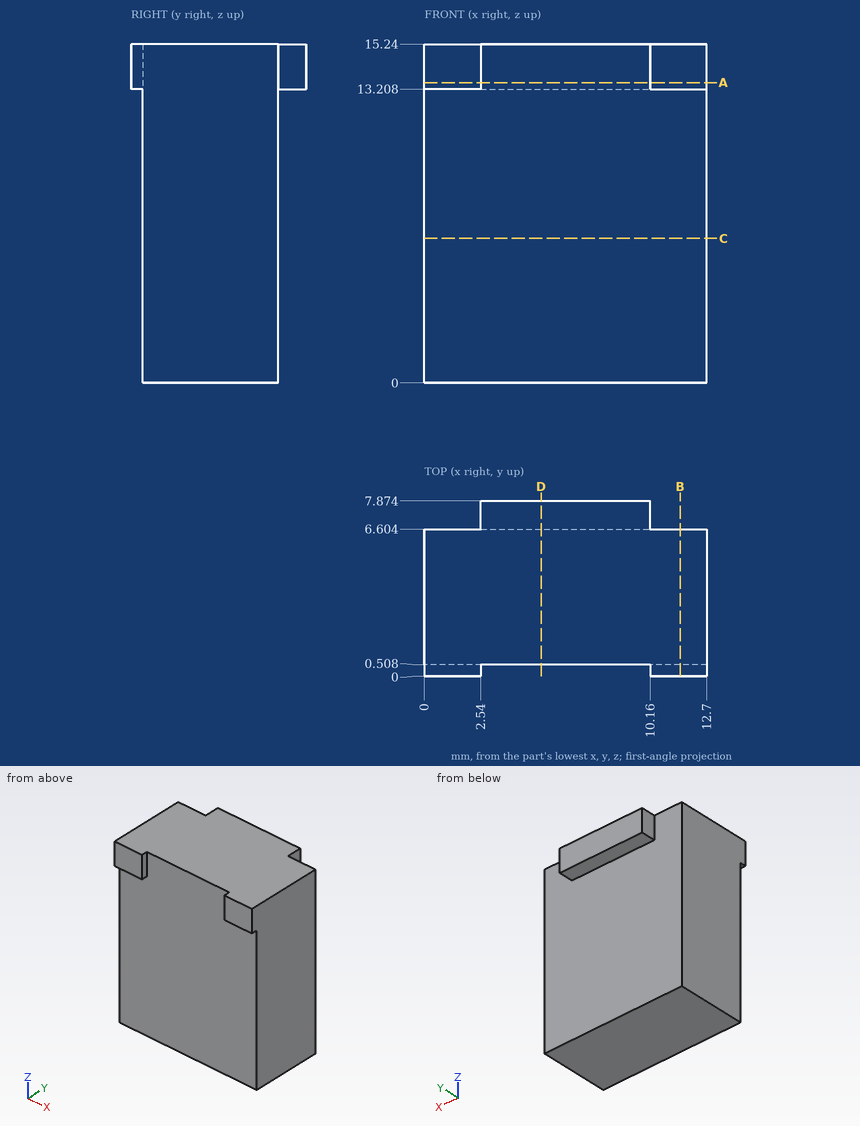
Verification items for this drawing (mm, ordinates from the low corner). Coordinates: 2 decimals unless noted, no trailing zeros. Loops run counter-clockwise (first coordinate to the right, second up) from the corner with the lowest first, then second, coordinate; pieces in that order, holes last. Notation, with made-up numbers: (18, 88) - (41, 88) arc R7 cw to (41, 97) - close; hole circle Ø4 at (26.25, 81). An arc over 180 degrees is marked (long way). One line per item, written item: value. Start each with the question number.
(1) Cross-section at D-D on x = 5.25. Enter the section's corners in (y, z).
(2) Cross-section at C-C on z = 6.5. Enter the section's corners in (x, y), plus the area to 3 significant figures.
(3) Cross-section at A-A on z = 13.5. Enter the section's corners in (x, y), plus the area to 3 significant figures.
(4) Depth check by flat-ended pin: P1, Ø0.6, axis at y = 7, z = 14, coming from the +X side; P2, Ø1, axis at x = 5.5, z = 9, coming from the -Y side; P3, Ø3, axis at x = 6.5, z = 2.5, coming from the +Y side. Enter the tip coordinate at first touch or a pass-through.
(5) Material ranges on line 1 (Y direction, x = 4, z = 10); line 2 (Y direction, x = 4.25, z = 13.25); line 3 (Z direction, x = 6, y = 7), recorded low to high. Write a range as [from, to].
(6) Cross-section at B-B on x = 11.5. Enter the section's corners in (y, z).
Results below:
1. outline: (0.51, 0) - (6.6, 0) - (6.6, 13.21) - (7.87, 13.21) - (7.87, 15.24) - (0.51, 15.24) - close
2. outline: (0, 0.51) - (12.7, 0.51) - (12.7, 6.6) - (0, 6.6) - close
2. area: 77.4 mm2
3. outline: (0, 0) - (2.54, 0) - (2.54, 0.51) - (10.16, 0.51) - (10.16, 0) - (12.7, 0) - (12.7, 6.6) - (10.16, 6.6) - (10.16, 7.87) - (2.54, 7.87) - (2.54, 6.6) - (0, 6.6) - close
3. area: 89.7 mm2
4. P1: stops at x = 10.16
4. P2: stops at y = 0.51
4. P3: stops at y = 6.6
5. line 1: y = [0.51, 6.6]
5. line 2: y = [0.51, 7.87]
5. line 3: z = [13.21, 15.24]
6. outline: (0, 13.21) - (0.51, 13.21) - (0.51, 0) - (6.6, 0) - (6.6, 15.24) - (0, 15.24) - close
